Geometry: final body of the model. Coordinates: model frame, mm. Face numbers are marked on the shaded views. Round coordinates to 2 decimals unless told otherwise and drop trailing zeros. Write each loop counter-clockwise with the first axis right and the second up, starting at its lowest first coordinate (ties: lowest second). Pieces come first, ordered by that corner, then holes. Notation, with made-up numbers: (-36.75, -8.5) -> (16.25, -8.5) arc R4 ccw to (16.25, -2.5) -> close; hole circle Ø1 at (-9, -19.75). An arc over 180 degrees is marked (long way). Use one line per item in the form item = value. Start each with the question number.
1. Draft query along Y for the marked faces 1, 2, 3 and 4. Return one class per face: pulls with the +Y half, pulls with the -Y half, needs draft (parallel to the pull), parting line crosses it, or undercut.
2. Cut plane D-D, the plane x = 6.35. Return the cut outline in (y, z) (3 decimals), plus the area to 3 significant figures.
3. Cut plane C-C, the plane z = 1.65. Return the cut outline in (x, y) (3 decimals), plus the area to 3 significant figures.
4. Pin query (flat end, axial travel): pin 1 Ø2 at (x, y) = (6.5, -8) entering from -Z; pin 2 Ø1.5 at (x, y) = (0, 1.75) entering from +Z. Return the tip coordinate at first contact, or that it passes through.
5. Line query: L1, parallel to Y at x = 0, z = 1.8; L2, parallel to X at y = 20.5, z = 1.1; L3, parallel to Y at x = -6.35, z = 1.65. Output: solid intervals per line, ascending.
6. Cut plane B-B, the plane y = -16. Return the cut outline in (x, z) (3 decimals).
7. Cut plane A-A, the plane y = 10.25. Return the cut outline in (x, z) (3 decimals), plus the area to 3 significant figures.
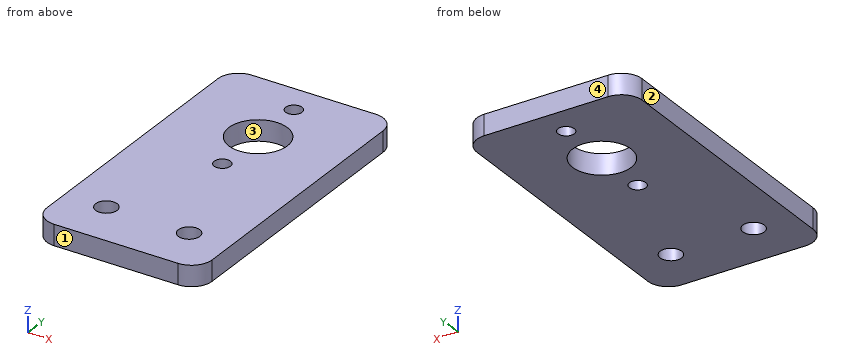
```python
from build123d import *

# Parameters (mm, degrees)
SKETCH1_W             = 25.4
SKETCH1_H             = 47
BOSS_EXTRUDE1_DEPTH   = 3.175
SKETCH2_R             = 4.5
CUT_EXTRUDE1_DEPTH    = 27.90019749
M3X0_5_TAPPED_HOLE1_D = 2.5
FILLET1_R             = 3.175
M4X0_7_TAPPED_HOLE1_D = 3.3


with BuildPart() as part:
    # Sketch1 → Boss-Extrude1 (new body)
    with BuildSketch(Plane.XY):
        Rectangle(SKETCH1_W, SKETCH1_H)
    extrude(amount=BOSS_EXTRUDE1_DEPTH)

    # Sketch2 → Cut-Extrude1 (cut, through all)
    with BuildSketch(Plane.XY.offset(3.175)):
        with Locations((0, 10.25)):
            Circle(SKETCH2_R)
    extrude(amount=-CUT_EXTRUDE1_DEPTH, mode=Mode.SUBTRACT)

    # M3x0.5 Tapped Hole1 (through all)
    with Locations(Plane.XY.offset(3.175)):
        with Locations((0, 18.75), (0, 1.75)):
            Hole(M3X0_5_TAPPED_HOLE1_D / 2)

    # Fillet1
    fillet1_edges = [part.edges().sort_by_distance(p)[0] for p in [
        (12.7, -23.5, 1.5875),
        (-12.7, -23.5, 1.5875),
        (-12.7, 23.5, 1.5875),
        (12.7, 23.5, 1.5875),
    ]]
    fillet(fillet1_edges, radius=FILLET1_R)

    # M4x0.7 Tapped Hole1 (through all)
    with Locations(Plane.XY.offset(3.175)):
        with Locations((-6.35, -16), (6.35, -16)):
            Hole(M4X0_7_TAPPED_HOLE1_D / 2)


solid = part.part
```
Outcome:
q1.face_1 = pulls with the -Y half
q1.face_2 = needs draft
q1.face_3 = undercut
q1.face_4 = pulls with the +Y half
q2.outline = (-23.5, 0) -> (-17.65, 0) -> (-17.65, 3.175) -> (-23.5, 3.175) -> close; (-14.35, 0) -> (23.5, 0) -> (23.5, 3.175) -> (-14.35, 3.175) -> close
q2.area = 139 mm^2
q3.outline = (-12.7, -20.325) arc R3.175 ccw to (-9.525, -23.5) -> (9.525, -23.5) arc R3.175 ccw to (12.7, -20.325) -> (12.7, 20.325) arc R3.175 ccw to (9.525, 23.5) -> (-9.525, 23.5) arc R3.175 ccw to (-12.7, 20.325) -> close; hole circle Ø3.3 at (-6.35, -16); hole circle Ø9 at (0, 10.25); hole circle Ø2.5 at (0, 1.75); hole circle Ø2.5 at (0, 18.75); hole circle Ø3.3 at (6.35, -16)
q3.area = 1,090 mm^2
q4.pin_1 = 0
q4.pin_2 = through
q5.L1 = -23.5 to 0.5, 3 to 5.75, 14.75 to 17.5, 20 to 23.5
q5.L2 = -12.7 to 12.7
q5.L3 = -23.5 to -17.65, -14.35 to 23.5
q6.outline = (-12.7, 0) -> (-8, 0) -> (-8, 3.175) -> (-12.7, 3.175) -> close; (-4.7, 0) -> (4.7, 0) -> (4.7, 3.175) -> (-4.7, 3.175) -> close; (8, 0) -> (12.7, 0) -> (12.7, 3.175) -> (8, 3.175) -> close
q7.outline = (-12.7, 0) -> (-4.5, 0) -> (-4.5, 3.175) -> (-12.7, 3.175) -> close; (4.5, 0) -> (12.7, 0) -> (12.7, 3.175) -> (4.5, 3.175) -> close
q7.area = 52.1 mm^2
